Verification items for the finished model (mm, model axes). A direction names the side the tool comes from. Round coordinates to 2 decimals unless told otherwise and drop trailing zeros. Order: outer loops, then holes, each group sorted by start corner. A loop starts at its lowest first (then second) coordinate and runs counter-clockwise, first axis right, second up. Notation, with made-up numbers: M 3.5,74.5 L 45.5,74.5 A22 cw 45.5,81.5 Z; hole C 51,61 d4. An arc over 180 degrees is marked long. One line per item, written item: value. Start each with the question number.
from build123d import *

# Parameters (mm, degrees)
SKETCH_1_R      = 2
SKETCH_1_W      = 4.2
SKETCH_1_H      = 8.2
SKETCH_1_R_2    = 1.5
SKETCH_1_R_3    = 5.03
EXTRUDE_1_DEPTH = 4


with BuildPart() as part:
    # 草图1 → 凸台-拉伸1 (new body)
    with BuildSketch(Plane.XY):
        with BuildLine():
            Line((0.838796757, -22.113571429), (-3.161203243, -22.113571429))
            Line((-3.161203243, -22.113571429), (-3.161203243, -31.344407284))
            Line((-3.161203243, -31.344407284), (-7.161203243, -31.344407284))
            Line((-7.161203243, -31.344407284), (-7.161203243, -39.344407284))
            Line((-7.161203243, -39.344407284), (-3.161203243, -39.344407284))
            Line((-3.161203243, -39.344407284), (11.838796757, -39.344407284))
            Line((11.838796757, -39.344407284), (115.338796757, 59.655592716))
            ThreePointArc((115.338796757, 59.655592716), (133.816387407, 87.309261363), (101.196661133, 93.797728339))
            Line((101.196661133, 93.797728339), (11.838796757, 49.807248516))
            Line((11.838796757, 49.807248516), (-3.161203243, 49.807248516))
            Line((-3.161203243, 49.807248516), (-3.161203243, 41.155592716))
            Line((-3.161203243, 41.155592716), (0.838796757, 41.155592716))
            Line((0.838796757, 41.155592716), (0.838796757, 42.505592716))
            Line((0.838796757, 42.505592716), (3.538796757, 42.505592716))
            Line((3.538796757, 42.505592716), (3.538796757, 41.155592716))
            Line((3.538796757, 41.155592716), (6.238796757, 41.155592716))
            Line((6.238796757, 41.155592716), (6.238796757, 38.155592716))
            Line((6.238796757, 38.155592716), (3.538796757, 38.155592716))
            Line((3.538796757, 38.155592716), (3.538796757, 36.805592716))
            Line((3.538796757, 36.805592716), (0.838796757, 36.805592716))
            Line((0.838796757, 36.805592716), (0.838796757, 38.155592716))
            Line((0.838796757, 38.155592716), (-3.161203243, 38.155592716))
            Line((-3.161203243, 38.155592716), (-3.161203243, 28.655592716))
            Line((-3.161203243, 28.655592716), (-7.161203243, 28.655592716))
            Line((-7.161203243, 28.655592716), (-7.161203243, 20.655592716))
            Line((-7.161203243, 20.655592716), (-3.161203243, 20.655592716))
            Line((-3.161203243, 20.655592716), (-3.161203243, 11.155592716))
            Line((-3.161203243, 11.155592716), (0.838796757, 11.155592716))
            Line((0.838796757, 11.155592716), (0.838796757, 12.505592716))
            Line((0.838796757, 12.505592716), (3.538796757, 12.505592716))
            Line((3.538796757, 12.505592716), (3.538796757, 11.155592716))
            Line((3.538796757, 11.155592716), (6.238796757, 11.155592716))
            Line((6.238796757, 11.155592716), (6.238796757, 8.155592716))
            Line((6.238796757, 8.155592716), (3.538796757, 8.155592716))
            Line((3.538796757, 8.155592716), (3.538796757, 6.805592716))
            Line((3.538796757, 6.805592716), (0.838796757, 6.805592716))
            Line((0.838796757, 6.805592716), (0.838796757, 8.155592716))
            Line((0.838796757, 8.155592716), (-3.161203243, 8.155592716))
            Line((-3.161203243, 8.155592716), (-3.161203243, -1.344407284))
            Line((-3.161203243, -1.344407284), (-7.161203243, -1.344407284))
            Line((-7.161203243, -1.344407284), (-7.161203243, -9.344407284))
            Line((-7.161203243, -9.344407284), (-3.161203243, -9.344407284))
            Line((-3.161203243, -9.344407284), (-3.161203243, -19.113571429))
            Line((-3.161203243, -19.113571429), (0.838796757, -19.113571429))
            Line((0.838796757, -19.113571429), (0.838796757, -17.763571429))
            Line((0.838796757, -17.763571429), (3.538796757, -17.763571429))
            Line((3.538796757, -17.763571429), (3.538796757, -19.113571429))
            Line((3.538796757, -19.113571429), (6.238796757, -19.113571429))
            Line((6.238796757, -19.113571429), (6.238796757, -22.113571429))
            Line((6.238796757, -22.113571429), (3.538796757, -22.113571429))
            Line((3.538796757, -22.113571429), (3.538796757, -23.463571429))
            Line((3.538796757, -23.463571429), (0.838796757, -23.463571429))
            Line((0.838796757, -23.463571429), (0.838796757, -22.113571429))
        make_face()
        with Locations((31.133984923, 26.166524095)):
            Circle(SKETCH_1_R, mode=Mode.SUBTRACT)
        with Locations((73.338796757, 37.976109285)):
            Rectangle(SKETCH_1_W, SKETCH_1_H, mode=Mode.SUBTRACT)
        with Locations((73.338796757, 52.976109285)):
            Circle(SKETCH_1_R_2, mode=Mode.SUBTRACT)
        with Locations((116.282857143, 79.386428571)):
            Circle(SKETCH_1_R_3, mode=Mode.SUBTRACT)
    extrude(amount=EXTRUDE_1_DEPTH)


solid = part.part
1. Section check A-A (z = 2.65). Give the number of separate pieces and of enclosed holes in the cut face, and give its area (3 significant figures).
2. Tool access check on faces 5 (the face through (-3.161, 46, 2)), 6 (the face through (73, 42.076, 2)), 7 (the face through (-1, -22.114, 2)). Record the directions out of +Z, -Z, +X, -X, +Y, -Y that give a thin tool (end or side, any length) a straight path to the whole face; none if there is none.
3. Draft check along Y on faces 1 (the face through (47, 31, 4)), 2 (the face through (-5, 28.656, 2)), 3 (the face through (-5, -1.344, 2)), 4 (the face through (-5, -9.344, 2)). Enter one of: released by +Y, released by -Y, zero draft, split by the parting line, or undercut.
4. Section check B-B (x = 89.5). Record the cut outline in (y, z).
5. Depth check by flat-ended pin: pin 1 (1.2 mm diameter, centred on x = -1, z = 2, fed in from +Y); pin 2 (5 mm diameter, centred on x = 71.5, y = 42.5, fed in from -Z); pin 3 (2 mm diameter, centred on y = 5.5, z = 2, fed in from -X). Enter the tip coordinate at first touch or a pass-through.
6. Scan lines: line 1 along Y through (x, z) = (1, 3.2); line 2 along Y through (x, z) = (116.5, 1.5); line 3 along Y through (x, z) = (11, 0.75). Record each from-to range of solid material in increasing order.
7. Section check C-C (y = -13). Record the cut outline in (x, z).
Geometry check:
1. separate pieces: 1
1. enclosed holes: 4
1. area: 8,570 mm²
2. face 5: +Z, -Z, -X, +Y
2. face 6: +Z, -Z
2. face 7: +Z, -Z, -X
3. face 1: zero draft
3. face 2: released by +Y
3. face 3: undercut
3. face 4: undercut
4. outline: M 34.94,0 L 88.04,0 L 88.04,4 L 34.94,4 Z
5. pin 1: stops at y = 49.81
5. pin 2: stops at z = 0
5. pin 3: stops at x = -3.16
6. line 1: y = -39.34 to -23.46, -17.76 to 6.81, 12.51 to 36.81, 42.51 to 49.81
6. line 2: y = 59.69 to 74.36, 84.41 to 99.62
6. line 3: y = -39.34 to 49.81
7. outline: M -3.16,0 L 39.38,0 L 39.38,4 L -3.16,4 Z
